Answer from the drawing. Dimensions are ordinates in mm from the lowest x, y and z of the part. A direction names the side the tool comes from. Give positions to 0.01 mm unless a question says otherwise; leave off trailing zeros. Loops run counter-clockwise (first coordinate to the right, second up) from the corner with the lowest first, then second, coordinate; pieces in that order, holes last. Notation, with made-up numbers: (67, 66.5) - (100, 66.5) arc R17 cw to (100, 80.5) - close; hole circle Ø10 at (-6.5, 68.25). An arc over 180 degrees is marked (long way). Put each result on its own line as item: value. Start each with the question number.
1. A cutting plane is placed at D-D, the plane x = 95. Determine the outline of the cut face in (y, z) (3 decimals).
2. Consider L1, parallel to Y at x = 77, z = 162; L2, parallel to X at y = 68, z = 35; L3, parallel to Z at x = 166, y = 10.5 (3 decimals). Determine where each line is inside the solid, lowest interval first. Write a range as from..to.
3. A cutting plane is placed at A-A, the plane x = 244.5. Determine the outline of the cut face in (y, z).
4. A cutting plane is placed at C-C, the plane y = 66.6. Determine the outline of the cut face in (x, z) (3 decimals), plus the area to 3 significant figures.
5. A cutting plane is placed at B-B, the plane z = 104.5. Determine the outline of the cut face in (x, y), plus the area to 3 significant figures.
6. For the marked faces 1, 2 and 3, determine the directions among +Z, -Z, +X, -X, +Y, -Y from which every point of the face is accessible in a straight line to the end or side of a thin tool.
7. Given pin 1 Ø10 at (x, z) = (144.5, 71) entering from -Y; pin 2 Ø10 at (x, y) = (188.5, 91.5) entering from -Z; pin 3 Ø0.5 at (y, z) = (81, 208) entering from -X, each flat-ended and moving along its own axis, determine where each tip first touches the part or whether it passes through.
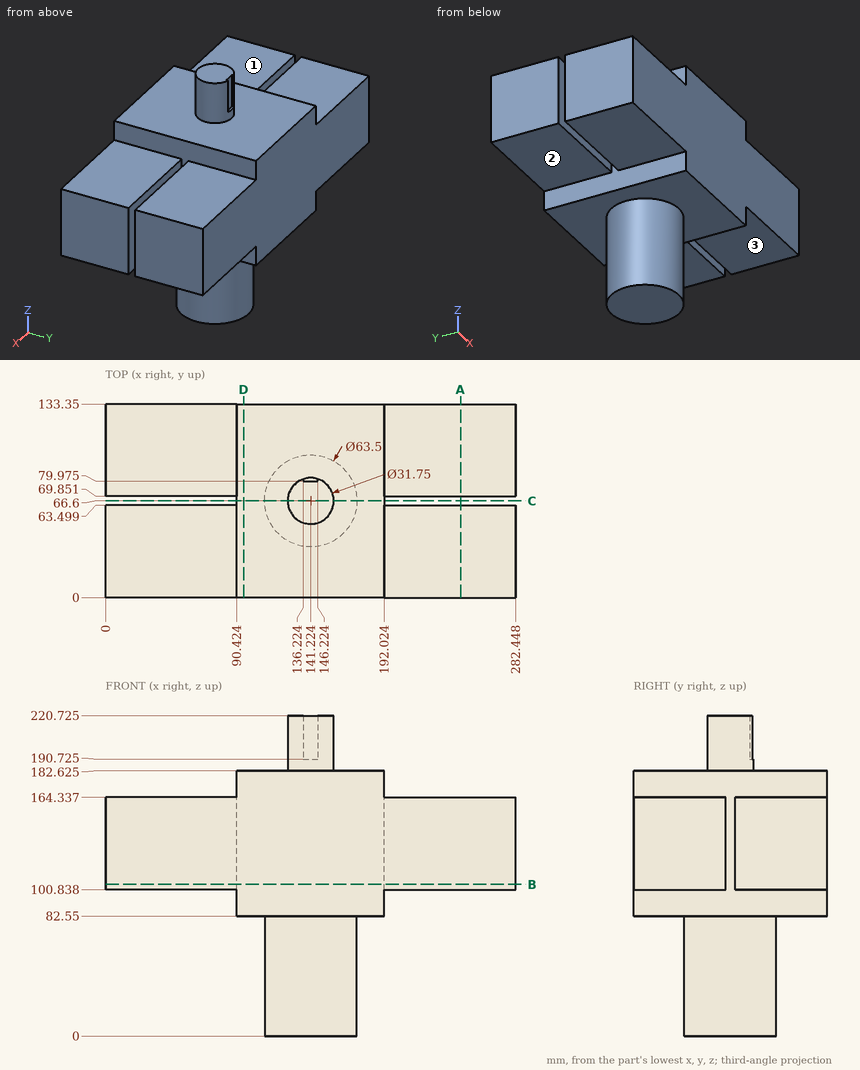
Return value:
1. outline: (0, 82.55) - (133.35, 82.55) - (133.35, 182.625) - (0, 182.625) - close
2. L1: y = 0..63.5, 69.85..133.35
2. L2: x = 109.5..172.94
2. L3: z = 82.55..182.625
3. outline: (0, 100.84) - (63.5, 100.84) - (63.5, 164.34) - (0, 164.34) - close; (69.85, 100.84) - (133.35, 100.84) - (133.35, 164.34) - (69.85, 164.34) - close
4. outline: (90.424, 82.55) - (109.474, 82.55) - (109.474, 0) - (172.974, 0) - (172.974, 82.55) - (192.024, 82.55) - (192.024, 182.625) - (157.099, 182.625) - (157.099, 220.725) - (125.349, 220.725) - (125.349, 182.625) - (90.424, 182.625) - close
4. area: 16,600 mm2
5. outline: (0, 0) - (282.45, 0) - (282.45, 63.5) - (192.02, 63.5) - (192.02, 69.85) - (282.45, 69.85) - (282.45, 133.35) - (0, 133.35) - (0, 69.85) - (90.42, 69.85) - (90.42, 63.5) - (0, 63.5) - close
5. area: 36,500 mm2
6. face 1: +Z, -X, +Y, -Y
6. face 2: -Z, -X, +Y, -Y
6. face 3: -Z, +X, +Y, -Y
7. pin 1: stops at y = 34.85
7. pin 2: stops at z = 82.55
7. pin 3: stops at x = 134.03
